Verification items for the finished model (mm, model axes). Face numbers are marked on the shaded views. A direction names the side the tool comes from. Give positions to 0.01 mm unless a question says otherwise; leave off trailing zeros. Loops run counter-clockwise (first coordinate to the right, second up) from the corner with the lowest first, then second, coordinate; pieces in that order, holes last. Notation, with made-up numbers: (23.25, 67.5) - (80.25, 67.5) arc R31 cw to (80.25, 95.5) - close; hole circle Ø10 at (29, 5). An arc over 180 degrees is marked (long way). One line per question, with ' | ' between items. Start each with the question number.
1. Thickness scan on line 1 along Y through (x, z) = (39.75, -1.55); line 2 along Y through (x, z) = (8, -3.4); line 3 along Y through (x, z) = (39, -2). Record the ranges inside material, lowest first. Write a range as from..to.
2. Mould release check, pull along Y, two halves, no side actions. Record for the marked faces 1, 2, 3 and 4: +Y half, -Y half, draft (parallel to the pull), parting line (faces both ways), or undercut.
3. Section check D-D, the plane y = 25. Enter the section's corners in (x, z).
4. Section check C-C, the plane z = 26.5. Enter the section's corners in (x, y).
5. Section check A-A, the plane x = 8. Enter the section's corners in (y, z), then the cut area to 3 significant figures.
6. Depth check by flat-ended pin: pin 1 Ø15 at (y, z) = (32, 2.5) entering from -X; pin 2 Ø5 at (x, y) = (25, 35) entering from +Z; pin 3 Ø3.5 at (x, y) = (-7, 35.5) entering from -Z; pin 4 Ø3 at (x, y) = (39.75, 14) entering from -Z. Enter the tip coordinate at first touch or a pass-through.
7. Tool access check on the marked faces 5, 6 and 7. Record the directions out of +Z, -Z, +X, -X, +Y, -Y that give a thin tool (end or side, any length) a straight path to the whole face; none if there is none.
8. Section check B-B, the plane y = 36. Enter the section's corners in (x, z).
from build123d import *

# Parameters (mm, degrees)
SKETCH1_W           = 55
SKETCH1_H           = 5
BOSS_EXTRUDE1_DEPTH = 50
SKETCH2_R           = 9.1
SKETCH2_R_2         = 1.6
CUT_EXTRUDE1_DEPTH  = 75.498322129
SKETCH3_W           = 5
SKETCH3_H           = 50
BOSS_EXTRUDE2_DEPTH = 30
SKETCH4_W           = 17
SKETCH4_H           = 50
BOSS_EXTRUDE3_DEPTH = 5


with BuildPart() as part:
    # Sketch1 → Boss-Extrude1 (new body)
    with BuildSketch(Plane(origin=(0, 0, 0), x_dir=(1, 0, 0), z_dir=(0, 1, 0))):
        with Locations((27.5, 2.5)):
            Rectangle(SKETCH1_W, SKETCH1_H)
    extrude(amount=BOSS_EXTRUDE1_DEPTH)

    # Sketch2 → Cut-Extrude1 (cut, through all)
    with BuildSketch(Plane.XY):
        with Locations((39.75, 25)):
            Circle(SKETCH2_R)
        with Locations((39.75, 36)):
            Circle(SKETCH2_R_2)
        with Locations((50.75, 25)):
            Circle(SKETCH2_R_2)
        with Locations((39.75, 14)):
            Circle(SKETCH2_R_2)
        with Locations((28.75, 25)):
            Circle(SKETCH2_R_2)
        with Locations((8, 40)):
            Circle(SKETCH2_R_2)
        with Locations((8, 10)):
            Circle(SKETCH2_R_2)
    extrude(amount=-CUT_EXTRUDE1_DEPTH, mode=Mode.SUBTRACT)

    # Sketch3 → Boss-Extrude2 (add)
    with BuildSketch(Plane.XY):
        with Locations((2.5, 25)):
            Rectangle(SKETCH3_W, SKETCH3_H)
    extrude(amount=BOSS_EXTRUDE2_DEPTH)

    # Sketch4 → Boss-Extrude3 (add)
    with BuildSketch(Plane.XY.offset(30)):
        with Locations((-3.5, 25)):
            Rectangle(SKETCH4_W, SKETCH4_H)
        with BuildLine():
            Line((-8, 46.6), (-3, 46.6))
            ThreePointArc((-3, 46.6), (-1.4, 45), (-3, 43.4))
            Line((-3, 43.4), (-8, 43.4))
            ThreePointArc((-8, 43.4), (-9.6, 45), (-8, 46.6))
        make_face(mode=Mode.SUBTRACT)
        with BuildLine():
            Line((-8, 3.4), (-3, 3.4))
            ThreePointArc((-3, 3.4), (-1.4, 5), (-3, 6.6))
            Line((-3, 6.6), (-8, 6.6))
            ThreePointArc((-8, 6.6), (-9.6, 5), (-8, 3.4))
        make_face(mode=Mode.SUBTRACT)
    extrude(amount=-BOSS_EXTRUDE3_DEPTH)


solid = part.part
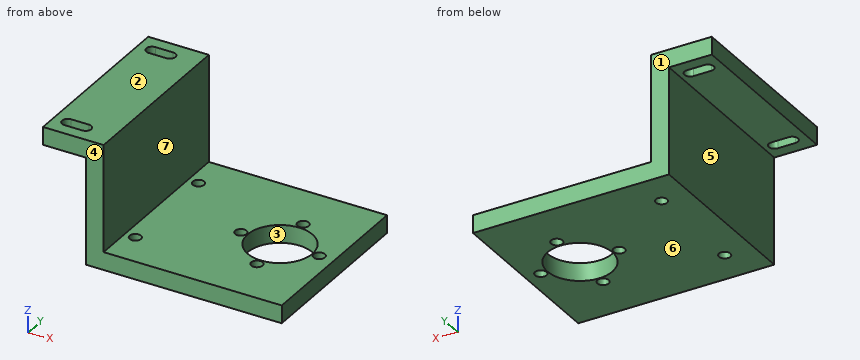
Results list:
1) line 1: 0..12.4, 15.6..15.9, 34.1..34.4, 37.6..50 | line 2: 0..8.4, 11.6..38.4, 41.6..50 | line 3: 0..12.59, 15.41..15.93, 34.07..34.59, 37.41..50
2) face 1: +Y half | face 2: draft | face 3: undercut | face 4: -Y half
3) outline: (-12, 25) - (0, 25) - (0, -5) - (27.15, -5) - (27.15, 0) - (5, 0) - (5, 30) - (-12, 30) - close; (30.35, -5) - (30.65, -5) - (30.65, 0) - (30.35, 0) - close; (48.85, -5) - (49.15, -5) - (49.15, 0) - (48.85, 0) - close; (52.35, -5) - (55, -5) - (55, 0) - (52.35, 0) - close
4) outline: (-12, 0) - (5, 0) - (5, 50) - (-12, 50) - close; hole (-8, 3.4) - (-3, 3.4) arc R1.6 ccw to (-3, 6.6) - (-8, 6.6) arc R1.6 ccw to start; hole (-8, 43.4) - (-3, 43.4) arc R1.6 ccw to (-3, 46.6) - (-8, 46.6) arc R1.6 ccw to start
5) outline: (0, -5) - (8.4, -5) - (8.4, 0) - (0, 0) - close; (11.6, -5) - (38.4, -5) - (38.4, 0) - (11.6, 0) - close; (41.6, -5) - (50, -5) - (50, 0) - (41.6, 0) - close | area: 218 mm²
6) pin 1: x = 0 | pin 2: z = 0 | pin 3: z = 25 | pin 4: through
7) face 5: -Z, -X, +Y, -Y | face 6: -Z, +X, -X, +Y, -Y | face 7: +Z, +X, +Y, -Y
8) outline: (-12, 25) - (0, 25) - (0, -5) - (38.15, -5) - (38.15, 0) - (5, 0) - (5, 30) - (-12, 30) - close; (41.35, -5) - (55, -5) - (55, 0) - (41.35, 0) - close
